The model under review builds one solid part; all positions refer to its coordinate system, in mm. A direction names the side the tool comes from. Coordinates: 2 decimals unless noted, no trailing zeros. Loops run counter-clockwise (first coordinate to the right, second up) from the corner with the lowest first, then second, coordinate; pieces in that order, holes last. Notation, with made-up numbers: M 37.25,17.5 L 48.25,17.5 A27 cw 48.25,36.5 Z; hole C -28,-34.5 d3. An arc over 180 degrees is marked long. One line per item, written item: value.
```python
from build123d import *

# Parameters (mm, degrees)
SKETCH_1_W               = 6.5
SKETCH_1_H               = 6.5
SKETCH_1_R               = 2.05
EXTRUDE_1_DEPTH          = 6.5
SKETCH_2_W               = 6.5
SKETCH_2_H               = 13
EXTRUDE_2_DEPTH          = 6.5
SKETCH_3_W               = 6.5
SKETCH_3_H               = 6.5
SKETCH_3_R               = 2.05
EXTRUDE_3_DEPTH          = 6.5
SKETCH_4_R               = 2.05
CUT_EXTRUDE_1_DEPTH      = 8
FILLET_1_R               = 3
FILLET_2_R               = 3
CUT_EXTRUDE_2_DEPTH      = 18.195428818
CUT_EXTRUDE_2_DEPTH_BACK = 18.195428818
SKETCH_5_W               = 7.542755484
SKETCH_5_H               = 3.936219418


with BuildPart() as part:
    # 草图1 → 凸台-拉伸1 (new body)
    with BuildSketch(Plane.XY):
        with Locations((-8.580694703, 4.782128964)):
            Rectangle(SKETCH_1_W, SKETCH_1_H)
        with Locations(Location((-8.580694703, 4.782128964, 0), (0, 0, 180))):
            Circle(SKETCH_1_R, mode=Mode.SUBTRACT)
    extrude(amount=EXTRUDE_1_DEPTH)

    # 草图2 → 凸台-拉伸2 (add)
    with BuildSketch(Plane(origin=(-5.330694703, 0, 0), x_dir=(0, 0, -1), z_dir=(1, 0, 0))):
        with Locations((3.25, 8.032128964)):
            Rectangle(SKETCH_2_W, SKETCH_2_H)
    extrude(amount=-EXTRUDE_2_DEPTH)

    # 草图3 → 凸台-拉伸3 (add)
    with BuildSketch(Plane(origin=(-5.330694703, 0, 0), x_dir=(0, 0, -1), z_dir=(1, 0, 0))):
        with Locations((3.25, 4.782128964)):
            Rectangle(SKETCH_3_W, SKETCH_3_H)
        with Locations(Location((3.25, 4.782128964, 0), (0, 0, 180))):
            Circle(SKETCH_3_R, mode=Mode.SUBTRACT)
    extrude(amount=EXTRUDE_3_DEPTH)

    # 草图4 → 切除-拉伸1 (cut)
    with BuildSketch(Plane(origin=(0, 14.532128964, 0), x_dir=(1, 0, 0), z_dir=(0, 1, 0))):
        with Locations(Location((-8.580694703, 3.25, 0), (0, 0, 270))):
            Circle(SKETCH_4_R)
    extrude(amount=-CUT_EXTRUDE_1_DEPTH, mode=Mode.SUBTRACT)

    # 圆角1
    fillet_1_edges = [part.edges().sort_by_distance(p)[0] for p in [
        (-5.330694703, 1.532128964, -6.5),
        (-11.830694703, 11.282128964, 0),
        (-11.830694703, 8.032128964, -6.5),
        (-5.330694703, 11.282128964, -6.5),
        (-2.080694703, 8.032128964, -6.5),
        (-11.830694703, 1.532128964, 0),
        (-11.830694703, 8.032128964, 3.25),
    ]]
    fillet(fillet_1_edges, radius=FILLET_1_R)

    # 圆角2
    # the kernel refuses this fillet: 3 mm, written as the material it adds along each edge
    with BuildSketch(Plane(origin=(-5.330694703, 1.532128964, 0), x_dir=(0, 0, 1), z_dir=(0, 1, 0))) as fillet_2_piece_1:
        with BuildLine():
            CenterArc((FILLET_2_R, FILLET_2_R), FILLET_2_R, 180, 90)
            Line((0, FILLET_2_R), (0, 0))
            Line((0, 0), (FILLET_2_R, 0))
        make_face()
    extrude(amount=6.5)

    # 草图5 → 切除-拉伸2 (cut, two sides: drawn at the far end of the back side and taken through both)
    with BuildSketch(Plane(origin=(-5.330694703, 0, 0), x_dir=(0, 0, -1), z_dir=(1, 0, 0)).offset(-CUT_EXTRUDE_2_DEPTH_BACK)):
        with Locations((3.771377742, 13.476899479)):
            Rectangle(SKETCH_5_W, SKETCH_5_H)
    extrude(amount=CUT_EXTRUDE_2_DEPTH + CUT_EXTRUDE_2_DEPTH_BACK, mode=Mode.SUBTRACT)


solid = part.part
```
(1) To check wall thickness, follow L1, parallel to X at y = 8.95, z = -3.25; L2, parallel to Y at x = -1, z = -3.25; L3, parallel to X at y = 7.8, z = -3.25. State the ranges of each line that lie inside material, in increasing order. Write a range as [from, to].
Checks:
L1: [-11.83, -10.63], [-6.53, -5.33]
L2: [1.53, 2.73], [6.83, 8.03]
L3: [-11.83, -10.63], [-6.53, 1.17]
(2) Insertion check: pin 1 Ø3 at (y, z) = (10, -1.5) entering from +X; pin 2 Ø1 at (x, y) = (-1, 4) entering from +Z; pin 3 Ø4 at (y, z) = (9, 5) entering from -X. Each pin has a flat end and moves straight along its axis. Give the tip position at first contact, or say it passes through.
Checks:
pin 1: x = -5.33
pin 2: z = 0
pin 3: x = -11.1
(3) Tool access review of faces 4 (the face through (-9, 6.532, -3)), 5 (the face through (-10.536, 4.166, 3.204)), 6 (the face through (-2.459, 7.177, -5.598)): name each direction out of +Z, -Z, +X, -X, +Y, -Y from which nothing blocks a thin tool from reaching the whole face with its end or side.
Checks:
face 4: +Y
face 5: +Z
face 6: -Z, +X, +Y
(4) Add section A-A on z = -3.25. State the section outline as (x, y) points, then the cut area to 3 significant figures.
Checks:
outline: M -11.83,4.53 A3 ccw -8.83,1.53 L 1.17,1.53 L 1.17,2.73 L -5.33,2.73 L -5.33,6.83 L 1.17,6.83 L 1.17,8.03 L -5.33,8.03 L -5.33,11.51 L -6.53,11.51 L -6.53,6.53 L -10.63,6.53 L -10.63,11.51 L -11.83,11.51 Z
area: 58.1 mm^2
(5) Add section C-C on z = 1.5. State the section outline as (x, y) points, then the cut area to 3 significant figures.
Checks:
outline: M -11.83,4.53 A3 ccw -8.83,1.53 L -4.93,1.53 L -4.93,8.03 L -8.83,8.03 A3 ccw -11.83,5.03 Z; hole C -8.58,4.78 d4.1
area: 27.8 mm^2
(6) Draft analysis for pull direction Z (two halves, no side actions). For faces 1 (the face through (-5.331, 5, -3)), 2 (the face through (-5.331, 10, -2)), 3 (the face through (-1, 5, 0)), state which applies: pulls with the +Z half, pulls with the -Z half, needs draft (parallel to the pull), parting line crosses it, or undercut.
Checks:
face 1: undercut
face 2: needs draft
face 3: pulls with the +Z half
(7) Add section D-D on x = -1.75. State the section outline as (y, z) points.
Checks:
outline: M 1.53,-3.5 A3 ccw 4.53,-6.5 L 5.03,-6.5 A3 ccw 8.03,-3.5 L 8.03,0 L 1.53,0 Z; hole C 4.78,-3.25 d4.1
(8) Add section B-B on y = 7.5. State the section outline as (x, z) points, then the cut area to 3 significant figures.
Checks:
outline: M -11.83,-3.5 A3 ccw -8.83,-6.5 L -8.33,-6.5 A3 ccw -5.86,-5.21 L 1.17,-5.21 L 1.17,0 L -2.33,0 A3 cw -5.33,3 L -5.33,6.5 L -10.54,6.5 L -10.54,-0.53 A3 ccw -11.83,-3 Z; hole C -8.58,-3.25 d4.1
area: 93.4 mm^2
